Print and shaded views of the part. All mm, measured from the part's lowest x, y and z. Give positions to 0.01 mm unless a question says otherwise; leave off trailing zeros. Loops run counter-clockwise (first coordinate to the right, second up) from the corner with the lowest first, then second, coordinate; pieces in that order, holes last.
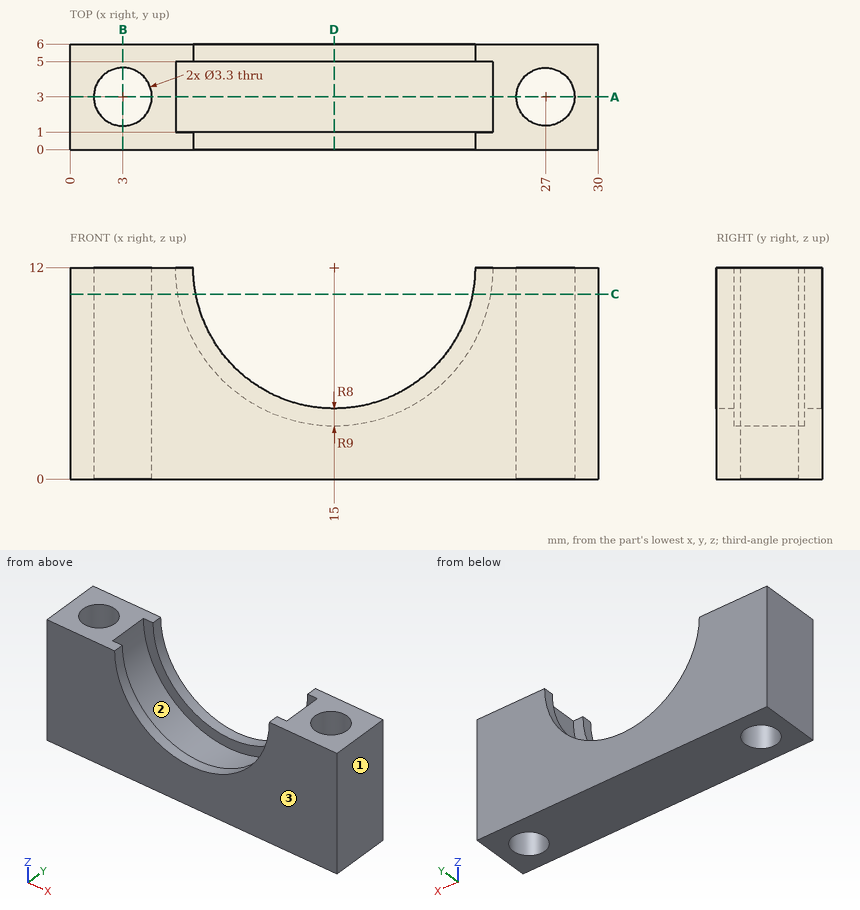
1. Probe line 1 along Y through (x, z) = (18, 4.5); line 2 along Y through (x, z) = (3, 9); line 3 along X through (y, z) = (3.7, 1). List the from-to ranges inside material, lowest first.
Responses:
line 1: y = 0 to 1, 5 to 6
line 2: y = 0 to 1.35, 4.65 to 6
line 3: x = 0 to 1.51, 4.49 to 25.51, 28.49 to 30
2. Saw through at B-B, the plane x = 3. List the corners of the cut face in (y, z).
Responses:
outline: (0, 0) - (1.35, 0) - (1.35, 12) - (0, 12) - close; (4.65, 0) - (6, 0) - (6, 12) - (4.65, 12) - close
3. Saw through at A-A, the plane y = 3. List the corners of the cut face in (x, z).
Responses:
outline: (0, 0) - (1.35, 0) - (1.35, 12) - (0, 12) - close; (4.65, 0) - (25.35, 0) - (25.35, 12) - (24, 12) arc R9 cw to (6, 12) - (4.65, 12) - close; (28.65, 0) - (30, 0) - (30, 12) - (28.65, 12) - close
4. Drop flat-ended pins along their axis: pin 1 (2 mm diameter, centred on x = 26, y = 3, fed in from +Z); pin 2 (3 mm diameter, centred on x = 27, y = 3, fed in from +Z). Give the stop position or say it passes through.
Responses:
pin 1: stops at z = 12
pin 2: passes through
5. Saw through at D-D, the plane x = 15. List the corners of the cut face in (y, z), and give its area (3 significant figures).
Responses:
outline: (0, 0) - (6, 0) - (6, 4) - (5, 4) - (5, 3) - (1, 3) - (1, 4) - (0, 4) - close
area: 20.0 mm2
6. Pull direction Y, two halves, no side cores. Call the marked faces 1, 2 and 3: released by +Y, released by -Y, zero draft, split by the parting line, or undercut.
Responses:
face 1: zero draft
face 2: undercut
face 3: released by -Y
7. Saw through at C-C, the plane z = 10.5. List the corners of the cut face in (x, y), and give its area (3 significant figures).
Responses:
outline: (0, 0) - (7.14, 0) - (7.14, 1) - (6.13, 1) - (6.13, 5) - (7.14, 5) - (7.14, 6) - (0, 6) - close; (22.86, 0) - (30, 0) - (30, 6) - (22.86, 6) - (22.86, 5) - (23.87, 5) - (23.87, 1) - (22.86, 1) - close; hole circle Ø3.3 at (3, 3); hole circle Ø3.3 at (27, 3)
area: 60.5 mm2
